```python
from build123d import *

# Parameters (mm, degrees)
BOSS_EXTRUDE1_DEPTH = 40
SKETCH3_W           = 12.7
SKETCH3_H           = 40
BOSS_EXTRUDE2_DEPTH = 27.178
SKETCH4_W           = 184.978795618
SKETCH4_H           = 131.733859804
CUT_EXTRUDE2_DEPTH  = 51
SKETCH5_W           = 144.166334374
SKETCH5_H           = 140.012963834
CUT_EXTRUDE3_DEPTH  = 18.25
SKETCH6_R           = 20
CUT_EXTRUDE4_DEPTH  = 20
FILLET4_R           = 3.175
SKETCH7_W           = 96.652193462
SKETCH7_H           = 93.586405028
CUT_EXTRUDE5_DEPTH  = 27.178
CUT_EXTRUDE6_DEPTH  = 41
CUT_EXTRUDE7_DEPTH  = 8
FILLET5_R           = 2
SKETCH10_R          = 1.75
CUT_EXTRUDE8_DEPTH  = 33.0000001
SKETCH11_W          = 9.551786503
SKETCH11_H          = 12
SKETCH11_W_2        = 7.9375
CUT_EXTRUDE9_DEPTH  = 19.05
SKETCH14_R          = 3
CUT_EXTRUDE10_DEPTH = 3.2
SKETCH15_W          = 61.098487026
SKETCH15_H          = 49.743772834
CUT_EXTRUDE11_DEPTH = 12.5


with BuildPart() as part:
    # Sketch1 → Boss-Extrude1 (new body)
    with BuildSketch(Plane(origin=(0, 0, 0), x_dir=(1, 0, 0), z_dir=(0, 1, 0))):
        with BuildLine():
            Line((-50, -50), (0, -50))
            Line((0, -50), (0, -30))
            ThreePointArc((0, -30), (-30, 0), (0, 30))
            Line((0, 30), (0, 50))
            Line((0, 50), (-50, 50))
            Line((-50, 50), (-50, -50))
        make_face()
        with BuildLine():
            Line((0, -30), (0, -50))
            Line((0, -50), (50, -50))
            Line((50, -50), (50, 50))
            Line((50, 50), (0, 50))
            Line((0, 50), (0, 30))
            ThreePointArc((0, 30), (21.213203436, 21.213203436), (30, 0))
            ThreePointArc((30, 0), (21.213203436, -21.213203436), (0, -30))
        make_face()
    extrude(amount=BOSS_EXTRUDE1_DEPTH)

    # Sketch3 → Boss-Extrude2 (add)
    with BuildSketch(Plane.XY.offset(50)):
        with Locations((-24.6, 20)):
            Rectangle(SKETCH3_W, SKETCH3_H)
    extrude(amount=BOSS_EXTRUDE2_DEPTH)

    # Sketch4 → Cut-Extrude2 (cut, through all)
    with BuildSketch(Plane(origin=(0, 0, 0), x_dir=(0, 0, -1), z_dir=(1, 0, 0))):
        Rectangle(SKETCH4_W, SKETCH4_H)
    extrude(amount=CUT_EXTRUDE2_DEPTH, mode=Mode.SUBTRACT)

    # Sketch5 → Cut-Extrude3 (cut)
    with BuildSketch(Plane(origin=(0, 0, 0), x_dir=(0, 0, -1), z_dir=(1, 0, 0))):
        Rectangle(SKETCH5_W, SKETCH5_H)
    extrude(amount=-CUT_EXTRUDE3_DEPTH, mode=Mode.SUBTRACT)

    # Sketch6 → Cut-Extrude4 (cut)
    with BuildSketch(Plane(origin=(0, 0, -50), x_dir=(-1, 0, 0), z_dir=(0, 0, -1))):
        with Locations((5.529693955, 22.14995336)):
            Circle(SKETCH6_R)
    extrude(amount=-CUT_EXTRUDE4_DEPTH, mode=Mode.SUBTRACT)

    # Fillet4
    fillet4_edges = [part.edges().sort_by_distance(p)[0] for p in [
        (-18.25, 6.716424466, -40),
        (-18.25, 37.583482255, -40),
    ]]
    fillet(fillet4_edges, radius=FILLET4_R)

    # Sketch7 → Cut-Extrude5 (cut)
    with BuildSketch(Plane.XY.offset(77.178)):
        Rectangle(SKETCH7_W, SKETCH7_H)
    extrude(amount=-CUT_EXTRUDE5_DEPTH, mode=Mode.SUBTRACT)

    # Sketch8 → Cut-Extrude6 (cut, through all)
    with BuildSketch(Plane(origin=(0, 40, 0), x_dir=(1, 0, 0), z_dir=(0, 1, 0))):
        with BuildLine():
            Line((-34.76, 50), (-50, 50))
            Line((-50, 50), (-50, -50))
            Line((-50, -50), (-34.125, -50))
            add(Edge.make_bspline(
                [(-34.125, -50), (-34.125, -33.241229213), (-45.237036485, -0.093705418), (-34.76, 33.330216103), (-34.76, 50)],
                knots=[0, 0, 0, 0, 0.500369617, 1, 1, 1, 1], degree=3))
        make_face()
    extrude(amount=-CUT_EXTRUDE6_DEPTH, mode=Mode.SUBTRACT)

    # Sketch9 → Cut-Extrude7 (cut)
    with BuildSketch(Plane(origin=(0, 40, 0), x_dir=(1, 0, 0), z_dir=(0, 1, 0))):
        with BuildLine():
            Line((-18.25, -50), (-18.25, -30.95))
            Line((-18.25, -30.95), (-35.932995014, -30.95))
            add(Edge.make_bspline(
                [(-34.125, -50), (-34.125, -43.629466822), (-34.928437006, -37.283896996), (-35.932995014, -30.95)],
                knots=[0, 0, 0, 0, 0.190206149, 0.190206149, 0.190206149, 0.190206149], degree=3))
            Line((-34.125, -50), (-18.25, -50))
        make_face()
    extrude(amount=-CUT_EXTRUDE7_DEPTH, mode=Mode.SUBTRACT)

    # Fillet5
    fillet5_edges = [part.edges().sort_by_distance(p)[0] for p in [
        (-27.091497507, 32, 30.95),
        (-27.091497507, 40, 30.95),
    ]]
    fillet(fillet5_edges, radius=FILLET5_R)

    # Sketch10 → Cut-Extrude8 (cut, through all)
    with BuildSketch(Plane(origin=(0, 32, 0), x_dir=(1, 0, 0), z_dir=(0, 1, 0))):
        with Locations((-26.1875, -46.5)):
            Circle(SKETCH10_R)
        with Locations((-26.1875, -36.5)):
            Circle(SKETCH10_R)
    extrude(amount=-CUT_EXTRUDE8_DEPTH, mode=Mode.SUBTRACT)

    # Sketch11 → Cut-Extrude9 (cut)
    with BuildSketch(Plane.XY.offset(50)):
        with Locations((-38.900893252, 16)):
            Rectangle(SKETCH11_W, SKETCH11_H)
        with Locations((-30.15625, 16)):
            Rectangle(SKETCH11_W_2, SKETCH11_H)
        with Locations((-22.21875, 16)):
            Rectangle(SKETCH11_W_2, SKETCH11_H)
    extrude(amount=-CUT_EXTRUDE9_DEPTH, mode=Mode.SUBTRACT)

    # Sketch14 → Cut-Extrude10 (cut)
    with BuildSketch(Plane(origin=(0, 32, 0), x_dir=(1, 0, 0), z_dir=(0, 1, 0))):
        with Locations((-26.1875, -36.5)):
            Circle(SKETCH14_R)
        with Locations((-26.1875, -46.5)):
            Circle(SKETCH14_R)
    cut_extrude10 = extrude(amount=-CUT_EXTRUDE10_DEPTH, mode=Mode.SUBTRACT)

    # Mirror2: Cut-Extrude10 across plane
    add(cut_extrude10.mirror(Plane.ZX.offset(16)), mode=Mode.SUBTRACT)

    # Sketch15 → Cut-Extrude11 (cut)
    with BuildSketch(Plane(origin=(0, 0, -50), x_dir=(-1, 0, 0), z_dir=(0, 0, -1))):
        with Locations((30.549243513, 24.871886417)):
            Rectangle(SKETCH15_W, SKETCH15_H)
    extrude(amount=-CUT_EXTRUDE11_DEPTH, mode=Mode.SUBTRACT)


solid = part.part
```
Geometry check sheet. Reference: the model listing, model coordinates, mm. A direction names the side the tool comes from. Give positions to 0.01 mm unless a question says otherwise; leave off trailing zeros. Write each question's results on one line, items separated by ' | '. Start each with the question number.
(1) Scan lines: line 1 (Y direction, x = -18.75, z = 34); line 2 (Z direction, x = -25.25, y = 27); line 3 (Z direction, x = -26.75, y = 4.5). Record each from-to range of solid material in increasing order.
(2) Gauge pin test, flat ends, axial feed: P1, Ø1.8, axis at x = -27, z = 35.5, coming from the +Y side; P2, Ø2, axis at y = 21.5, z = -2.5, coming from the +X side; P3, Ø3, axis at x = -23.5, y = 37, coming from the +Z side. Record the tip position at first contact, or that the pin passes through.
(3) Mould release check, pull along Z, two halves, no side actions. Record for faces 6 (the face through (-21, 22, -30)), 7 (the face through (-18.517, 6.56, -33.802)), 8 (the face through (-25, 28.8, 38)): pulls with the +Z half, pulls with the -Z half, needs draft (parallel to the pull), parting line crosses it, or undercut.
(4) Access from +Z, -Z, +X, -X, +Y, -Y to the whole of each face (thin tool, end or side, straight path). Record for faces 1 (the face through (-25, 3.2, 38)), 2 (the face through (-27.58, 6.65, 37.56)), 3 (the face through (-28.399, 30.422, 34.472)), 4 (the face through (-27, 22, 41)), 5 (the face through (-27, 32, 41)).
(5) Sectioned sample at A-A (y = 26.5). Give the number of separate pieces and of enclosed holes in the cut face, plus the area to 3 significant figures.
Answer below:
1) line 1: 0 to 10, 22 to 32 | line 2: -37.5 to -16.2, 16.2 to 35.02, 37.98 to 45.02, 47.98 to 50 | line 3: -37.5 to -13.58, 13.58 to 34.84, 38.16 to 44.84, 48.16 to 50
2) P1: y = 28.8 | P2: x = -29.8 | P3: z = 30.95
3) face 6: pulls with the -Z half | face 7: needs draft | face 8: undercut
4) face 1: -Y | face 2: +Y, -Y | face 3: +Y | face 4: +Z, +X, -X | face 5: +Z, +X, -X, +Y
5) separate pieces: 1 | enclosed holes: 2 | area: 1,220 mm2
